Can you work these out from the model? Positions are in its coordinate system, mm. Give positions to 0.01 mm unless a question says otherwise; leave off trailing zeros. Order: outer loops, then holes, each group sorted by start corner. A loop starts at its lowest first (then second) coordinate and runs counter-clockwise, first axis right, second up. Notation, with made-up numbers: M 18,45 L 56,45 A31 cw 56,79 Z; hole C 39.5,18.25 d9. An arc over 180 degrees is marked long. Answer as a JSON object with one key per item and string values.
```python
from build123d import *

# Parameters (mm, degrees)
F0_R     = 3.846045
F1_DEPTH = 10


with BuildPart() as f1:
    # F0 (on Top) → F1 (new body)
    with BuildSketch(Plane.XY):
        with BuildLine():
            Line((-37.795966, 13.42895), (-15.622052, 13.42895))
            Line((-15.622052, 13.42895), (-15.622052, 23.42895))
            ThreePointArc((-15.622052, 23.42895), (-18.550985, 30.500018), (-25.622052, 33.42895))
            Line((-25.622052, 33.42895), (-37.795966, 33.42895))
            Line((-37.795966, 33.42895), (-37.795966, 13.42895))
        make_face()
        with Locations((-26.709009, 23.42895)):
            Circle(F0_R, mode=Mode.SUBTRACT)
    extrude(amount=F1_DEPTH)


solid = f1.part
```
1) I want a section at A-A on x = -26.25. Write out the boundary of the cut face in (y, z).
Results found:
{"outline": "M 13.43,0 L 19.61,0 L 19.61,10 L 13.43,10 Z; M 27.25,0 L 33.43,0 L 33.43,10 L 27.25,10 Z"}
2) I want a section at C-C on z = 3.5. Write out the boundary of the cut face in (x, y), and give its area (3 significant figures).
Results found:
{"outline": "M -37.8,13.43 L -15.62,13.43 L -15.62,23.43 A10 ccw -25.62,33.43 L -37.8,33.43 Z; hole C -26.71,23.43 d7.69", "area": "376 mm²"}
3) I'm going to push flat-ended pins straight in: pin 1 Ø7 at (x, y) = (-26.71, 23.43) entering from -Z; pin 2 Ø6 at (y, z) = (26, 8) entering from +X. Where does each tip first touch, or does it pass through?
Results found:
{"pin 1": "passes through", "pin 2": "stops at x = -15.62"}
4) I want a section at D-D on x = -21.25. Write out the boundary of the cut face in (y, z).
Results found:
{"outline": "M 13.43,0 L 32.42,0 L 32.42,10 L 13.43,10 Z"}
5) Thinking about a two-plate mould opening in X: for faces 1 (the face through (-18.47, 30.42, 4.93)), 2 (the face through (-30.55, 23.6, 4.93)), 3 (the face through (-27, 19, 0)), which applies, pulls with the +X half, pulls with the -X half, needs draft (parallel to the pull), parting line crosses it, or undercut?
Results found:
{"face 1": "pulls with the +X half", "face 2": "undercut", "face 3": "needs draft"}
6) I need wall thicknesses on L1, parallel to X at y = 21, z = 6; L2, parallel to X at y = 22.25, z = 1; L3, parallel to Y at x = -29, z = 2.25. Which ranges of each line are inside material? Lowest first, please.
Results found:
{"L1": "x = -37.8 to -29.69, -23.73 to -15.62", "L2": "x = -37.8 to -30.37, -23.05 to -15.62", "L3": "y = 13.43 to 20.34, 26.52 to 33.43"}
7) I want a section at B-B on y = 26. Write out the boundary of the cut face in (x, z).
Results found:
{"outline": "M -37.8,0 L -29.57,0 L -29.57,10 L -37.8,10 Z; M -23.85,0 L -15.96,0 L -15.96,10 L -23.85,10 Z"}
